from build123d import *

# Parameters (mm, degrees)
BOSS_EXTRUDE1_DEPTH = 250
SKETCH2_R           = 3.4
CUT_EXTRUDE1_DEPTH  = 251.898385806
FILLET1_R           = 2.5
FILLET2_R           = 0.25
SKETCH3_R           = 3.4
BOSS_EXTRUDE3_DEPTH = 250


with BuildPart() as part:
    # Sketch1 → Boss-Extrude1 (new body)
    with BuildSketch(Plane.XY):
        Polygon((-15, 15), (-5.2, 15), (-5.2, 13.808325472), (-4.1, 13.808325472), (-4.1, 12.8), (-8.25, 12.8), (-8.25, 9.664213562), (-4.385786438, 5.8), (4.385786438, 5.8), (8.25, 9.664213562), (8.25, 12.8), (4.1, 12.8), (4.1, 13.808325472), (5.2, 13.808325472), (5.2, 15), (15, 15), (15, 5.2), (13.808325472, 5.2), (13.808325472, 4.1), (12.8, 4.1), (12.8, 8.25), (9.664213562, 8.25), (5.8, 4.385786438), (5.8, -4.385786438), (9.664213562, -8.25), (12.8, -8.25), (12.8, -4.1), (13.808325472, -4.1), (13.808325472, -5.2), (15, -5.2), (15, -15), (5.2, -15), (5.2, -13.808325472), (4.1, -13.808325472), (4.1, -12.8), (8.25, -12.8), (8.25, -9.664213562), (4.385786438, -5.8), (-4.385786438, -5.8), (-8.25, -9.664213562), (-8.25, -12.8), (-4.1, -12.8), (-4.1, -13.808325472), (-5.2, -13.808325472), (-5.2, -15), (-15, -15), (-15, -5.2), (-13.808325472, -5.2), (-13.808325472, -4.1), (-12.8, -4.1), (-12.8, -8.25), (-9.664213562, -8.25), (-5.8, -4.385786438), (-5.8, 4.385786438), (-9.664213562, 8.25), (-12.8, 8.25), (-12.8, 4.1), (-13.808325472, 4.1), (-13.808325472, 5.2), (-15, 5.2), align=None)
    extrude(amount=BOSS_EXTRUDE1_DEPTH)

    # Sketch2 → Cut-Extrude1 (cut, through all)
    with BuildSketch(Plane.XY.offset(250)):
        Circle(SKETCH2_R)
        with BuildLine():
            Line((-12.5, 13.5), (-10.5, 13.5))
            ThreePointArc((-10.5, 13.5), (-9.792893219, 13.207106781), (-9.5, 12.5))
            Line((-9.5, 12.5), (-9.5, 10.5))
            ThreePointArc((-9.5, 10.5), (-9.792893219, 9.792893219), (-10.5, 9.5))
            Line((-10.5, 9.5), (-12.5, 9.5))
            ThreePointArc((-12.5, 9.5), (-13.207106781, 9.792893219), (-13.5, 10.5))
            Line((-13.5, 10.5), (-13.5, 12.5))
            ThreePointArc((-13.5, 12.5), (-13.207106781, 13.207106781), (-12.5, 13.5))
        make_face()
        with BuildLine():
            Line((9.5, 12.5), (9.5, 10.5))
            ThreePointArc((9.5, 10.5), (9.792893219, 9.792893219), (10.5, 9.5))
            Line((10.5, 9.5), (12.5, 9.5))
            ThreePointArc((12.5, 9.5), (13.207106781, 9.792893219), (13.5, 10.5))
            Line((13.5, 10.5), (13.5, 12.5))
            ThreePointArc((13.5, 12.5), (13.207106781, 13.207106781), (12.5, 13.5))
            Line((12.5, 13.5), (10.5, 13.5))
            ThreePointArc((10.5, 13.5), (9.792893219, 13.207106781), (9.5, 12.5))
        make_face()
        with BuildLine():
            Line((12.5, -13.5), (10.5, -13.5))
            ThreePointArc((10.5, -13.5), (9.792893219, -13.207106781), (9.5, -12.5))
            Line((9.5, -12.5), (9.5, -10.5))
            ThreePointArc((9.5, -10.5), (9.792893219, -9.792893219), (10.5, -9.5))
            Line((10.5, -9.5), (12.5, -9.5))
            ThreePointArc((12.5, -9.5), (13.207106781, -9.792893219), (13.5, -10.5))
            Line((13.5, -10.5), (13.5, -12.5))
            ThreePointArc((13.5, -12.5), (13.207106781, -13.207106781), (12.5, -13.5))
        make_face()
        with BuildLine():
            Line((-9.5, -12.5), (-9.5, -10.5))
            ThreePointArc((-9.5, -10.5), (-9.792893219, -9.792893219), (-10.5, -9.5))
            Line((-10.5, -9.5), (-12.5, -9.5))
            ThreePointArc((-12.5, -9.5), (-13.207106781, -9.792893219), (-13.5, -10.5))
            Line((-13.5, -10.5), (-13.5, -12.5))
            ThreePointArc((-13.5, -12.5), (-13.207106781, -13.207106781), (-12.5, -13.5))
            Line((-12.5, -13.5), (-10.5, -13.5))
            ThreePointArc((-10.5, -13.5), (-9.792893219, -13.207106781), (-9.5, -12.5))
        make_face()
    extrude(amount=-CUT_EXTRUDE1_DEPTH, mode=Mode.SUBTRACT)

    # Fillet1
    fillet1_edges = [part.edges().sort_by_distance(p)[0] for p in [
        (15, -15, 125),
        (-15, -15, 125),
        (-15, 15, 125),
        (15, 15, 125),
    ]]
    fillet(fillet1_edges, radius=FILLET1_R)

    # Fillet2
    fillet2_edges = [part.edges().sort_by_distance(p)[0] for p in [
        (5.2, -15, 125),
        (5.2, -13.808325472, 125),
        (4.1, -13.808325472, 125),
        (-4.1, -13.808325472, 125),
        (-5.2, -13.808325472, 125),
        (-5.2, -15, 125),
        (-15, -5.2, 125),
        (-13.808325472, -5.2, 125),
        (-13.808325472, -4.1, 125),
        (-13.808325472, 4.1, 125),
        (-13.808325472, 5.2, 125),
        (-15, 5.2, 125),
        (-5.2, 15, 125),
        (-5.2, 13.808325472, 125),
        (-4.1, 13.808325472, 125),
        (4.1, 13.808325472, 125),
        (5.2, 13.808325472, 125),
        (5.2, 15, 125),
        (15, 5.2, 125),
        (13.808325472, 5.2, 125),
        (13.808325472, 4.1, 125),
        (13.808325472, -4.1, 125),
        (13.808325472, -5.2, 125),
        (15, -5.2, 125),
    ]]
    fillet(fillet2_edges, radius=FILLET2_R)

    # Sketch3 → Boss-Extrude3 (add)
    with BuildSketch(Plane(origin=(0, 0, 0), x_dir=(-1, 0, 0), z_dir=(0, 0, -1))):
        with BuildLine():
            Line((12.8, 4.1), (13.558325472, 4.1))
            ThreePointArc((13.558325472, 4.1), (13.735102167, 4.173223305), (13.808325472, 4.35))
            Line((13.808325472, 4.35), (13.808325472, 4.95))
            ThreePointArc((13.808325472, 4.95), (13.881548777, 5.126776695), (14.058325472, 5.2))
            Line((14.058325472, 5.2), (14.75, 5.2))
            ThreePointArc((14.75, 5.2), (14.926776695, 5.273223305), (15, 5.45))
            Line((15, 5.45), (15, 12.5))
            ThreePointArc((15, 12.5), (14.267766953, 14.267766953), (12.5, 15))
            Line((12.5, 15), (5.45, 15))
            ThreePointArc((5.45, 15), (5.273223305, 14.926776695), (5.2, 14.75))
            Line((5.2, 14.75), (5.2, 14.058325472))
            ThreePointArc((5.2, 14.058325472), (5.126776695, 13.881548777), (4.95, 13.808325472))
            Line((4.95, 13.808325472), (4.35, 13.808325472))
            ThreePointArc((4.35, 13.808325472), (4.173223305, 13.735102167), (4.1, 13.558325472))
            Line((4.1, 13.558325472), (4.1, 12.8))
            Line((4.1, 12.8), (8.25, 12.8))
            Line((8.25, 12.8), (8.25, 9.664213562))
            Line((8.25, 9.664213562), (4.385786438, 5.8))
            Line((4.385786438, 5.8), (-4.385786438, 5.8))
            Line((-4.385786438, 5.8), (-8.25, 9.664213562))
            Line((-8.25, 9.664213562), (-8.25, 12.8))
            Line((-8.25, 12.8), (-4.1, 12.8))
            Line((-4.1, 12.8), (-4.1, 13.558325472))
            ThreePointArc((-4.1, 13.558325472), (-4.173223305, 13.735102167), (-4.35, 13.808325472))
            Line((-4.35, 13.808325472), (-4.95, 13.808325472))
            ThreePointArc((-4.95, 13.808325472), (-5.126776695, 13.881548777), (-5.2, 14.058325472))
            Line((-5.2, 14.058325472), (-5.2, 14.75))
            ThreePointArc((-5.2, 14.75), (-5.273223305, 14.926776695), (-5.45, 15))
            Line((-5.45, 15), (-12.5, 15))
            ThreePointArc((-12.5, 15), (-14.267766953, 14.267766953), (-15, 12.5))
            Line((-15, 12.5), (-15, 5.45))
            ThreePointArc((-15, 5.45), (-14.926776695, 5.273223305), (-14.75, 5.2))
            Line((-14.75, 5.2), (-14.058325472, 5.2))
            ThreePointArc((-14.058325472, 5.2), (-13.881548777, 5.126776695), (-13.808325472, 4.95))
            Line((-13.808325472, 4.95), (-13.808325472, 4.35))
            ThreePointArc((-13.808325472, 4.35), (-13.735102167, 4.173223305), (-13.558325472, 4.1))
            Line((-13.558325472, 4.1), (-12.8, 4.1))
            Line((-12.8, 4.1), (-12.8, 8.25))
            Line((-12.8, 8.25), (-9.664213562, 8.25))
            Line((-9.664213562, 8.25), (-5.8, 4.385786438))
            Line((-5.8, 4.385786438), (-5.8, -4.385786438))
            Line((-5.8, -4.385786438), (-9.664213562, -8.25))
            Line((-9.664213562, -8.25), (-12.8, -8.25))
            Line((-12.8, -8.25), (-12.8, -4.1))
            Line((-12.8, -4.1), (-13.558325472, -4.1))
            ThreePointArc((-13.558325472, -4.1), (-13.735102167, -4.173223305), (-13.808325472, -4.35))
            Line((-13.808325472, -4.35), (-13.808325472, -4.95))
            ThreePointArc((-13.808325472, -4.95), (-13.881548777, -5.126776695), (-14.058325472, -5.2))
            Line((-14.058325472, -5.2), (-14.75, -5.2))
            ThreePointArc((-14.75, -5.2), (-14.926776695, -5.273223305), (-15, -5.45))
            Line((-15, -5.45), (-15, -12.5))
            ThreePointArc((-15, -12.5), (-14.267766953, -14.267766953), (-12.5, -15))
            Line((-12.5, -15), (-5.45, -15))
            ThreePointArc((-5.45, -15), (-5.273223305, -14.926776695), (-5.2, -14.75))
            Line((-5.2, -14.75), (-5.2, -14.058325472))
            ThreePointArc((-5.2, -14.058325472), (-5.126776695, -13.881548777), (-4.95, -13.808325472))
            Line((-4.95, -13.808325472), (-4.35, -13.808325472))
            ThreePointArc((-4.35, -13.808325472), (-4.173223305, -13.735102167), (-4.1, -13.558325472))
            Line((-4.1, -13.558325472), (-4.1, -12.8))
            Line((-4.1, -12.8), (-8.25, -12.8))
            Line((-8.25, -12.8), (-8.25, -9.664213562))
            Line((-8.25, -9.664213562), (-4.385786438, -5.8))
            Line((-4.385786438, -5.8), (4.385786438, -5.8))
            Line((4.385786438, -5.8), (8.25, -9.664213562))
            Line((8.25, -9.664213562), (8.25, -12.8))
            Line((8.25, -12.8), (4.1, -12.8))
            Line((4.1, -12.8), (4.1, -13.558325472))
            ThreePointArc((4.1, -13.558325472), (4.173223305, -13.735102167), (4.35, -13.808325472))
            Line((4.35, -13.808325472), (4.95, -13.808325472))
            ThreePointArc((4.95, -13.808325472), (5.126776695, -13.881548777), (5.2, -14.058325472))
            Line((5.2, -14.058325472), (5.2, -14.75))
            ThreePointArc((5.2, -14.75), (5.273223305, -14.926776695), (5.45, -15))
            Line((5.45, -15), (12.5, -15))
            ThreePointArc((12.5, -15), (14.267766953, -14.267766953), (15, -12.5))
            Line((15, -12.5), (15, -5.45))
            ThreePointArc((15, -5.45), (14.926776695, -5.273223305), (14.75, -5.2))
            Line((14.75, -5.2), (14.058325472, -5.2))
            ThreePointArc((14.058325472, -5.2), (13.881548777, -5.126776695), (13.808325472, -4.95))
            Line((13.808325472, -4.95), (13.808325472, -4.35))
            ThreePointArc((13.808325472, -4.35), (13.735102167, -4.173223305), (13.558325472, -4.1))
            Line((13.558325472, -4.1), (12.8, -4.1))
            Line((12.8, -4.1), (12.8, -8.25))
            Line((12.8, -8.25), (9.664213562, -8.25))
            Line((9.664213562, -8.25), (5.8, -4.385786438))
            Line((5.8, -4.385786438), (5.8, 4.385786438))
            Line((5.8, 4.385786438), (9.664213562, 8.25))
            Line((9.664213562, 8.25), (12.8, 8.25))
            Line((12.8, 8.25), (12.8, 4.1))
        make_face()
        with Locations(Location((0, 0, 0), (0, 0, 180))):
            Circle(SKETCH3_R, mode=Mode.SUBTRACT)
        with BuildLine():
            Line((-9.5, 12.5), (-9.5, 10.5))
            ThreePointArc((-9.5, 10.5), (-9.792893219, 9.792893219), (-10.5, 9.5))
            Line((-10.5, 9.5), (-12.5, 9.5))
            ThreePointArc((-12.5, 9.5), (-13.207106781, 9.792893219), (-13.5, 10.5))
            Line((-13.5, 10.5), (-13.5, 12.5))
            ThreePointArc((-13.5, 12.5), (-13.207106781, 13.207106781), (-12.5, 13.5))
            Line((-12.5, 13.5), (-10.5, 13.5))
            ThreePointArc((-10.5, 13.5), (-9.792893219, 13.207106781), (-9.5, 12.5))
        make_face(mode=Mode.SUBTRACT)
        with BuildLine():
            Line((12.5, 9.5), (10.5, 9.5))
            ThreePointArc((10.5, 9.5), (9.792893219, 9.792893219), (9.5, 10.5))
            Line((9.5, 10.5), (9.5, 12.5))
            ThreePointArc((9.5, 12.5), (9.792893219, 13.207106781), (10.5, 13.5))
            Line((10.5, 13.5), (12.5, 13.5))
            ThreePointArc((12.5, 13.5), (13.207106781, 13.207106781), (13.5, 12.5))
            Line((13.5, 12.5), (13.5, 10.5))
            ThreePointArc((13.5, 10.5), (13.207106781, 9.792893219), (12.5, 9.5))
        make_face(mode=Mode.SUBTRACT)
        with BuildLine():
            Line((9.5, -12.5), (9.5, -10.5))
            ThreePointArc((9.5, -10.5), (9.792893219, -9.792893219), (10.5, -9.5))
            Line((10.5, -9.5), (12.5, -9.5))
            ThreePointArc((12.5, -9.5), (13.207106781, -9.792893219), (13.5, -10.5))
            Line((13.5, -10.5), (13.5, -12.5))
            ThreePointArc((13.5, -12.5), (13.207106781, -13.207106781), (12.5, -13.5))
            Line((12.5, -13.5), (10.5, -13.5))
            ThreePointArc((10.5, -13.5), (9.792893219, -13.207106781), (9.5, -12.5))
        make_face(mode=Mode.SUBTRACT)
        with BuildLine():
            Line((-9.5, -10.5), (-9.5, -12.5))
            ThreePointArc((-9.5, -12.5), (-9.792893219, -13.207106781), (-10.5, -13.5))
            Line((-10.5, -13.5), (-12.5, -13.5))
            ThreePointArc((-12.5, -13.5), (-13.207106781, -13.207106781), (-13.5, -12.5))
            Line((-13.5, -12.5), (-13.5, -10.5))
            ThreePointArc((-13.5, -10.5), (-13.207106781, -9.792893219), (-12.5, -9.5))
            Line((-12.5, -9.5), (-10.5, -9.5))
            ThreePointArc((-10.5, -9.5), (-9.792893219, -9.792893219), (-9.5, -10.5))
        make_face(mode=Mode.SUBTRACT)
    extrude(amount=BOSS_EXTRUDE3_DEPTH)


solid = part.part
Here's how the part is built. I have some questions about the finished solid (model axes, mm). Give positions to 0.01 mm unless a question says otherwise; leave off trailing zeros. One line per item, written item: value. Start each with the question number.
1. We'd pull the mould along X, two halves only. Please class faces 1 (the face through (3.4, -1.04, -250)), 2 (the face through (0, 5.8, 4)): released by +X, released by -X, zero draft, split by the parting line, or undercut.
2. Imagine slicing it at A-A, the plane z = -212.5. Count the separate pieces of the cut face and the enclosed holes in it, plus the area to 3 significant figures.
3. I need wall thicknesses on probe 1 along X at (y, z) = (-12, -80); probe 2 along Y at (x, z) = (-6.25, -159); probe 3 along X at (y, z) = (0, -69.5). Which ranges of each line are inside material? Lowest first, please. Write a range as from..to.
4. Will these pins go through, and if not, where does the flat tip stop? pin 1 Ø1.5 at (x, z) = (0, 34) entering from -Y; pin 2 Ø5 at (y, z) = (0, -29.5) entering from +X; pin 3 Ø0.8 at (y, z) = (-14.5, 44.5) entering from -X.
Values follow:
1. face 1: zero draft
1. face 2: undercut
2. separate pieces: 1
2. enclosed holes: 5
2. area: 313 mm2
3. probe 1: x = -15..-13.5, -9.5..-8.25, 8.25..9.5, 13.5..15
3. probe 2: y = -15..-12.8, -7.66..-4.84, 4.84..7.66, 12.8..15
3. probe 3: x = -5.8..-3.4, 3.4..5.8
4. pin 1: stops at y = -5.8
4. pin 2: stops at x = 5.8
4. pin 3: stops at x = -14.42
